Can you work these out from the model? Positions are in its coordinate system, mm. A direction names the side the tool comes from. Coordinates: 2 decimals unless noted, no trailing zeros. Order: outer loops, then holes, each group sorted by start corner. A loop starts at its lowest first (then second) coordinate and runs counter-clockwise, first axis right, second up. Notation, with made-up numbers: (-17, 78) -> (2, 78) arc R17 ccw to (2, 87) -> close; hole circle Ø4 at (45, -33.75). An arc over 180 degrees is marked (long way). Answer in a Markdown table with one row per item. Add a question column.
1. Imagine slicing it at B-B on z = 2.65. State how many separate pieces and enclosed holes the cut face has, plus the area to 3 significant figures.
2. If I drill on line 1 along Y through (x, z) = (0, 1.75) (3 decimals); line 2 along Y through (x, z) = (50.8, 2.4) (3 decimals); line 3 along X through (y, z) = (-23, 1.4), over which ranges is the centre line in solid material (lowest first)? Write a range as [from, to].
3. Imagine slicing it at C-C on y = 0. Write out the boundary of the cut face in (x, z) (3 decimals).
4. Imagine slicing it at D-D on x = 15.5. Write out the boundary of the cut face in (y, z) (3 decimals).
5. On a 3-axis mill with a long thin cutter (end or side, diameter ignored), from which of +Z, -Z, +X, -X, +Y, -Y can I reach the whole of each face in a straight line? I mean faces 1 (the face through (35.59, -36.25, 1.57)), 2 (the face through (-34, -28.575, 2)). Say none if no direction works.
6. Imagine slicing it at A-A on x = 0. Write out the boundary of the cut face in (y, z) (3 decimals).
7. Will these pins go through, and if not, where does the flat tip stop? pin 1 (1.6 mm diameter, centred on y = -24.5, z = 2.5, fed in from +X); pin 2 (1.6 mm diameter, centred on y = 26, z = 1.5, fed in from +X); pin 3 (1.6 mm diameter, centred on x = -34.5, z = 1.5, fed in from -Y).
8. We'd pull the mould along Y, two halves only. Please class faces 3 (the face through (-57.15, 0.15, 1.57)), 4 (the face through (34, -28.575, 2)), 5 (the face through (36.25, 35.59, 1.57)), 6 (the face through (-32.643, -25, 2)): pulls with the +Y half, pulls with the -Y half, needs draft (parallel to the pull), parting line crosses it, or undercut.
from build123d import *

# Parameters (mm, degrees)
F0_W     = 3.175
F0_H     = 6.35
F0_R     = 1.905
F0_R_2   = 1.524
F1_DEPTH = 3.175


# Not quite as in the source:
# - a length typed as a fraction of an inch, garbled in the dataset ("3 / 203.2 mm" for 3/8 in), is restored


with BuildPart() as f1:
    # F0 (on Top) → F1 (new body)
    with BuildSketch(Plane.XY):
        with BuildLine():
            ThreePointArc((-50.403125, 6.3375855209), (-57.15, 0), (-50.403125, -6.3375855209))
            ThreePointArc((-50.403125, -6.3375855209), (-35.9210244843, -35.9210244843), (-6.3375855209, -50.403125))
            ThreePointArc((-6.3375855209, -50.403125), (0, -57.15), (6.3375855209, -50.403125))
            ThreePointArc((6.3375855209, -50.403125), (35.9210244843, -35.9210244843), (50.403125, -6.3375855209))
            ThreePointArc((50.403125, -6.3375855209), (57.15, 0), (50.403125, 6.3375855209))
            ThreePointArc((50.403125, 6.3375855209), (35.9210244843, 35.9210244843), (6.3375855209, 50.403125))
            ThreePointArc((6.3375855209, 50.403125), (0, 57.15), (-6.3375855209, 50.403125))
            ThreePointArc((-6.3375855209, 50.403125), (-35.9210244843, 35.9210244843), (-50.403125, 6.3375855209))
        make_face()
        with Locations((-34.2304483056, -25.4)):
            Rectangle(F0_W, F0_H, mode=Mode.SUBTRACT)
        with Locations((0, -50.8)):
            Circle(F0_R, mode=Mode.SUBTRACT)
        with Locations((34.2304483056, -25.4)):
            Rectangle(F0_W, F0_H, mode=Mode.SUBTRACT)
        with Locations((-50.8, 0)):
            Circle(F0_R, mode=Mode.SUBTRACT)
        with Locations((-34.2304483056, 0)):
            Circle(F0_R_2, mode=Mode.SUBTRACT)
        with Locations((-34.2304483056, 25.4)):
            Rectangle(F0_W, F0_H, mode=Mode.SUBTRACT)
        with Locations((34.2304483056, 0)):
            Circle(F0_R_2, mode=Mode.SUBTRACT)
        with Locations((50.8, 0)):
            Circle(F0_R, mode=Mode.SUBTRACT)
        with Locations((34.2304483056, 25.4)):
            Rectangle(F0_W, F0_H, mode=Mode.SUBTRACT)
        with Locations((0, 50.8)):
            Circle(F0_R, mode=Mode.SUBTRACT)
    extrude(amount=F1_DEPTH)


solid = f1.part
Answers follow:
| question | item | result |
|---|---|---|
| 1 | separate pieces | 1 |
| 1 | enclosed holes | 10 |
| 1 | area | 8,230 mm² |
| 2 | line 1 | y = [-57.15, -52.705], [-48.895, 48.895], [52.705, 57.15] |
| 2 | line 2 | y = [-6.35, -1.905], [1.905, 6.35] |
| 2 | line 3 | x = [-45.3, -35.82], [-32.64, 32.64], [35.82, 45.3] |
| 3 | outline | (-57.15, 0) -> (-52.705, 0) -> (-52.705, 3.175) -> (-57.15, 3.175) -> close; (-48.895, 0) -> (-35.754, 0) -> (-35.754, 3.175) -> (-48.895, 3.175) -> close; (-32.706, 0) -> (32.706, 0) -> (32.706, 3.175) -> (-32.706, 3.175) -> close; (35.754, 0) -> (48.895, 0) -> (48.895, 3.175) -> (35.754, 3.175) -> close; (52.705, 0) -> (57.15, 0) -> (57.15, 3.175) -> (52.705, 3.175) -> close |
| 4 | outline | (-48.378, 0) -> (48.378, 0) -> (48.378, 3.175) -> (-48.378, 3.175) -> close |
| 5 | face 1 | +Z, -Z, +X, -Y |
| 5 | face 2 | +Z, -Z |
| 6 | outline | (-57.15, 0) -> (-52.705, 0) -> (-52.705, 3.175) -> (-57.15, 3.175) -> close; (-48.895, 0) -> (48.895, 0) -> (48.895, 3.175) -> (-48.895, 3.175) -> close; (52.705, 0) -> (57.15, 0) -> (57.15, 3.175) -> (52.705, 3.175) -> close |
| 7 | pin 1 | stops at x = 44.93 |
| 7 | pin 2 | stops at x = 44.11 |
| 7 | pin 3 | stops at y = -38.01 |
| 8 | face 3 | parting line crosses it |
| 8 | face 4 | undercut |
| 8 | face 5 | pulls with the +Y half |
| 8 | face 6 | undercut |
